Geometry: final body of the model. Coordinates: model frame, mm. Give positions to 0.01 mm unless a question says otherwise; leave off trailing zeros. Loops run counter-clockwise (first coordinate to the right, second up) from the corner with the lowest first, then second, coordinate; pieces in that order, holes last. Notation, with made-up numbers: (23, 54.5) -> (34, 54.5) arc R24 cw to (34, 75.5) -> close; hole circle Ø10 at (66.5, 7.25). An arc over 180 degrees is marked (long way). Answer in a Markdown table with one row per item. Add a question column.
1) Section query B-B (y = 0.6). Return the cut outline in (x, z).
2) Section query A-A (z = 0). Return the cut outline in (x, y).
3) Draft query along X for faces 1 (the flat face through (0, 0, 0)), 2 (the cylindrical face through (2.4, 2, 0.1)), 3 (the cylindrical face through (1.846, 1.037, 3.549)). Return one class per face: +X half, -X half, draft (parallel to the pull), parting line (faces both ways), or undercut.
4) First-contact query: P1, Ø1, axis at y = 1, z = -1.5, coming from the +X side. Flat tip, straight axial feed; report the tip coordinate or a pass-through.
5) Line query: line 1 (Z direction, x = 3, y = 1.6); line 2 (Y direction, x = -1.25, z = 2.5). Output: solid intervals per line, ascending. Write a range as from..to.
```python
from build123d import *

# Parameters (mm, degrees)
SKETCH_1_R          = 4
EXTRUDE_1_DEPTH     = 2
CUT_EXTRUDE_1_DEPTH = 4
CHAMFER_1_SIZE      = 0.1


with BuildPart() as part:
    # 草图1 → 凸台-拉伸1 (new body)
    with BuildSketch(Plane(origin=(0, 0, 0), x_dir=(1, 0, 0), z_dir=(0, 1, 0))):
        Circle(SKETCH_1_R)
    extrude(amount=EXTRUDE_1_DEPTH)

    # 草图2 → 切除-拉伸1 (cut, symmetric)
    with BuildSketch(Plane.XY):
        with BuildLine():
            Line((-4.460903823, 1.508767734), (-4.68289812, 3.453905247))
            Line((-4.68289812, 3.453905247), (4.900344987, 2.697866633))
            Line((4.900344987, 2.697866633), (4.2, 1.8))
            ThreePointArc((4.2, 1.8), (3.6, 2), (3, 1.8))
            ThreePointArc((3, 1.8), (2.4, 2), (1.8, 1.8))
            ThreePointArc((1.8, 1.8), (1.2, 2), (0.6, 1.8))
            ThreePointArc((0.6, 1.8), (0, 2), (-0.6, 1.8))
            ThreePointArc((-0.6, 1.8), (-1.2, 2), (-1.8, 1.8))
            ThreePointArc((-1.8, 1.8), (-2.4, 2), (-3, 1.8))
            ThreePointArc((-3, 1.8), (-3.79550386, 1.980702932), (-4.460903823, 1.508767734))
        make_face()
    extrude(amount=CUT_EXTRUDE_1_DEPTH, both=True, mode=Mode.SUBTRACT)

    # 倒角1
    chamfer_1_edges = [part.edges().sort_by_distance(p)[0] for p in [
        (-4, 0, 0),
    ]]
    chamfer(chamfer_1_edges, length=CHAMFER_1_SIZE)


solid = part.part
```
Evaluation:
| question | item | result |
|---|---|---|
| 1 | outline | circle Ø8 at (0, 0) |
| 2 | outline | (-4, 0.1) -> (-3.9, 0) -> (3.9, 0) -> (4, 0.1) -> (4, 1.92) arc R1 ccw to (3, 1.8) arc R1 ccw to (1.8, 1.8) arc R1 ccw to (0.6, 1.8) arc R1 ccw to (-0.6, 1.8) arc R1 ccw to (-1.8, 1.8) arc R1 ccw to (-3, 1.8) arc R1 ccw to (-4, 1.92) -> close |
| 3 | face 1 | draft |
| 3 | face 2 | undercut |
| 3 | face 3 | parting line |
| 4 | P1 | x = 3.87 |
| 5 | line 1 | -2.65..2.65 |
| 5 | line 2 | 0..2 |
